Drawing for the job (mm, zero at the part's lowest x, y, z). A direction names the side the tool comes from. Coordinates: 2 decimals unless noted, no trailing zeros. Write each loop counter-clockwise with the first axis right and the second up, starting at its lowest first coordinate (ties: lowest second). Pieces come first, ordered by that corner, then holes. Notation, with made-up numbers: M 4.5,71.25 L 31.5,71.25 A16 ccw 31.5,87.25 Z; hole C -8.5,19 d11. An arc over 180 degrees is marked long. Put each result on its own line as item: value. Start each with the question number.
Q1. Cut at C-C (y = 10.2). Write the cut outline in (x, z) (1 decimal), then the cut area to 3 significant figures.
Q2. Cut at A-A (x = 10.2). Write the cut outline in (y, z) (1 decimal).
Q3. Which spindle directions (+Z, -Z, +X, -X, +Y, -Y) get a long thin tool onto all of the face, cutting with end or side? Do the marked faces 1 and 2. Say none if no direction does.
Q4. Drill centre lines: line 1 along Z through (x, y) = (49, 10.5) (1 decimal); line 2 along X through (y, z) = (11.25, 6) (1 decimal); line 3 along Y through (x, z) = (55, 5.5). Where is each one in solid material? Low to high.
Q5. Cut at D-D (x = 57.5). Write the cut outline in (y, z) (1 decimal), then the cut area to 3 significant figures.
Q6. Cut at B-B (z = 5.5). Write the cut outline in (x, y) (1 decimal).
Q7. Drop flat-ended pins along their axis: pin 1 (2 mm diameter, centred on x = 36, y = 7, fed in from -Z) (1 decimal); pin 2 (1 mm diameter, centred on x = 47.5, z = 6, fed in from -Y); pin 3 (2 mm diameter, centred on y = 6.5, z = 3, fed in from -X); pin 4 (3 mm diameter, centred on x = 17.5, y = 6, fed in from +Z) (1 decimal). Give the stop position or say it passes through.
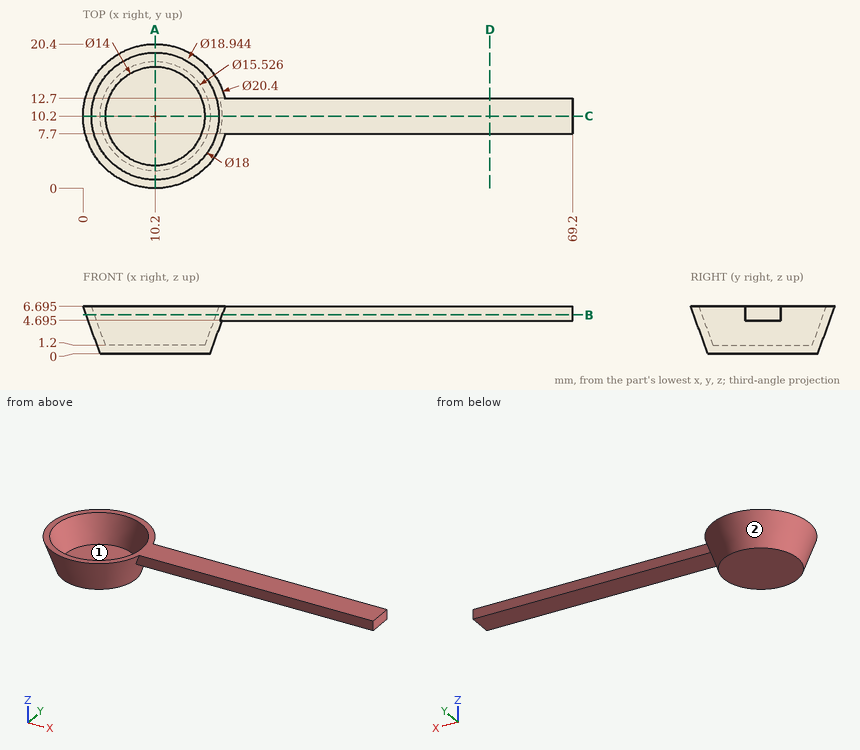
Computed values:
1. outline: M 0,6.7 L 2.4,0 L 18,0 L 19.7,4.7 L 69.2,4.7 L 69.2,6.7 L 19.2,6.7 L 17.2,1.2 L 3.2,1.2 L 1.2,6.7 Z
1. area: 131 mm2
2. outline: M 0,6.7 L 2.4,0 L 18,0 L 20.4,6.7 L 19.2,6.7 L 17.2,1.2 L 3.2,1.2 L 1.2,6.7 Z
3. face 1: +Z
3. face 2: -Z
4. line 1: 4.7 to 6.7
4. line 2: 0.3 to 1.5, 18.9 to 69.2
4. line 3: 7.7 to 12.7
5. outline: M 7.7,4.7 L 12.7,4.7 L 12.7,6.7 L 7.7,6.7 Z
5. area: 10.0 mm2
6. outline: M 19.6,7.7 L 69.2,7.7 L 69.2,12.7 L 19.6,12.7 A9.8 ccw long Z; hole C 10.2,10.2 d17.1
7. pin 1: z = 4.7
7. pin 2: y = 7.7
7. pin 3: x = 1.59
7. pin 4: z = 6.7
